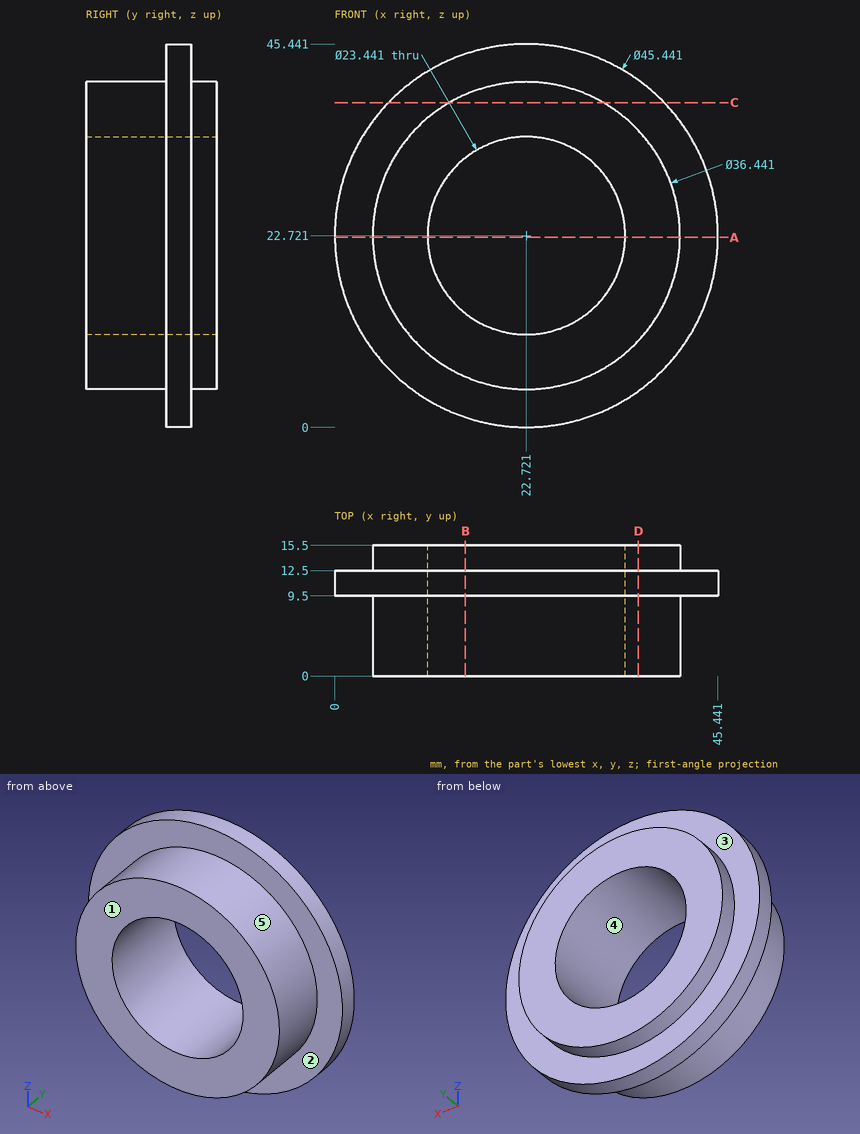
Check sheet for the drawn part. Datum: minimum x, y, z corner. Units: mm. A direction names the side the tool comes from. Coordinates: 2 decimals unless noted, no trailing zeros. Loops run counter-clockwise (first coordinate to the right, second up) from the corner with the lowest first, then second, coordinate; pieces in that order, holes last. Notation, with made-up numbers: (84, 67) -> (143, 67) arc R26 ccw to (143, 96) -> close; hole circle Ø7 at (-20.5, 43.25). An arc over 180 degrees is marked (long way). Write each question's results on one line, items separated by ' | '.
Item 1: Mould release check, pull along Z, two halves, no side actions. Record for the marked faces 3, 4 and 5: +Z half, -Z half, draft (parallel to the pull), parting line (faces both ways), or undercut.
Found:
face 3: draft | face 4: undercut | face 5: parting line
Item 2: Section check C-C, the plane z = 38.5. Enter the section's corners in (x, y).
Found:
outline: (6.37, 9.5) -> (13.61, 9.5) -> (13.61, 0) -> (31.83, 0) -> (31.83, 9.5) -> (39.07, 9.5) -> (39.07, 12.5) -> (31.83, 12.5) -> (31.83, 15.5) -> (13.61, 15.5) -> (13.61, 12.5) -> (6.37, 12.5) -> close
Item 3: Section check B-B, the plane x = 15.5. Enter the section's corners in (y, z), plus the area to 3 significant figures.
Found:
outline: (0, 5.99) -> (9.5, 5.99) -> (9.5, 1.18) -> (12.5, 1.18) -> (12.5, 5.99) -> (15.5, 5.99) -> (15.5, 13.49) -> (0, 13.49) -> close; (0, 31.95) -> (15.5, 31.95) -> (15.5, 39.45) -> (12.5, 39.45) -> (12.5, 44.26) -> (9.5, 44.26) -> (9.5, 39.45) -> (0, 39.45) -> close | area: 261 mm2
Item 4: Tool access check on the marked faces 1 and 2. Record the directions out of +Z, -Z, +X, -X, +Y, -Y that give a thin tool (end or side, any length) a straight path to the whole face; none if there is none.
Found:
face 1: +Z, -Z, +X, -X, -Y | face 2: -Y
Item 5: Section check A-A, the plane z = 22.5. Enter the section's corners in (x, y).
Found:
outline: (0, 9.5) -> (4.5, 9.5) -> (4.5, 0) -> (11, 0) -> (11, 15.5) -> (4.5, 15.5) -> (4.5, 12.5) -> (0, 12.5) -> close; (34.44, 0) -> (40.94, 0) -> (40.94, 9.5) -> (45.44, 9.5) -> (45.44, 12.5) -> (40.94, 12.5) -> (40.94, 15.5) -> (34.44, 15.5) -> close
Item 6: Material ranges on L1, parallel to Y at x = 11, z = 4.5; L2, parallel to X at y = 2.5, z = 29 (1 decimal); L3, parallel to X at y = 3, z = 30 (1 decimal), recorded low to high.
Found:
L1: y = 9.5 to 12.5 | L2: x = 5.6 to 12.8, 32.6 to 39.8 | L3: x = 6 to 13.5, 31.9 to 39.4
Item 7: Section check D-D, the plane x = 36. Enter the section's corners in (y, z) (1 decimal).
Found:
outline: (0, 10.2) -> (9.5, 10.2) -> (9.5, 4.3) -> (12.5, 4.3) -> (12.5, 10.2) -> (15.5, 10.2) -> (15.5, 35.2) -> (12.5, 35.2) -> (12.5, 41.2) -> (9.5, 41.2) -> (9.5, 35.2) -> (0, 35.2) -> close
Item 8: Gauge pin test, flat ends, axial feed: pin 1 (2 mm diameter, centred on x = 28.5, z = 14.5, fed in from -Y); pin 2 (6 mm diameter, centred on x = 38.5, y = 9.5, fed in from +Z) (1 decimal); pin 3 (6 mm diameter, centred on x = 33, y = 13, fed in from +Z); pin 4 (2 mm diameter, centred on x = 39.5, z = 12.5, fed in from -Y). Record the tip position at first contact, or that the pin passes through.
Found:
pin 1: passes through | pin 2: stops at z = 41.5 | pin 3: stops at z = 44.23 | pin 4: stops at y = 9.5
